Work out the finished part from the listing and answer in its coordinate system (mm). A direction names the side the tool comes from. Round coordinates to 2 decimals unless told otherwise and drop trailing zeros. Loops run counter-clockwise (first coordinate to the right, second up) from the corner with the lowest first, then second, coordinate; pieces in that order, holes last.
```python
from build123d import *

# Parameters (mm, degrees)
F0_R      = 23.300807
F1_DEPTH  = 76.2
F3_R      = 50.8
F3_R_2    = 23.300807
F4_DEPTH  = 12.7
F6_R      = 50.8
F6_R_2    = 23.300807
F7_DEPTH  = 12.7
F8_R      = 23.300807
F8_R_2    = 19.05
F9_DEPTH  = 12.7
F10_R     = 23.300807
F10_R_2   = 19.05
F11_DEPTH = 12.7
F12_R     = 6.35
F13_DEPTH = 2540


with BuildPart() as f1:
    # F0 (on Right) → F1 (new body)
    with BuildSketch(Plane.YZ):
        Circle(F0_R)
    extrude(amount=F1_DEPTH)



with BuildPart() as f4:
    # F3 (on face) → F4 (new body)
    with BuildSketch(Plane(origin=(0, 0, 0), x_dir=(0, -1, 0), z_dir=(-1, 0, 0))):
        Circle(F3_R)
        Circle(F3_R_2, mode=Mode.SUBTRACT)
    extrude(amount=F4_DEPTH)


with BuildPart() as f7:
    # F6 (on face) → F7 (new body)
    with BuildSketch(Plane.YZ.offset(76.2)):
        Circle(F6_R)
        Circle(F6_R_2, mode=Mode.SUBTRACT)
    extrude(amount=F7_DEPTH)


with BuildPart() as f1_1:
    add(f1.part)

    add(f7.part)  # F9 merges F7
    # F8 (on face) → F9 (join)
    with BuildSketch(Plane.YZ.offset(76.2)):
        Circle(F8_R)
        Circle(F8_R_2, mode=Mode.SUBTRACT)
    extrude(amount=F9_DEPTH)


    add(f4.part)  # F11 merges F4
    # F10 (on face) → F11 (join)
    with BuildSketch(Plane(origin=(0, 0, 0), x_dir=(0, -1, 0), z_dir=(-1, 0, 0))):
        Circle(F10_R)
        Circle(F10_R_2, mode=Mode.SUBTRACT)
    extrude(amount=F11_DEPTH)

    # F12 (on face) → F13 (cut)
    with BuildSketch(Plane(origin=(-12.7, 0, 0), x_dir=(0, -1, 0), z_dir=(-1, 0, 0))):
        with Locations((-38.1, 12.7)):
            Circle(F12_R)
        with Locations((-38.1, -12.7)):
            Circle(F12_R)
        with Locations((38.1, -12.7)):
            Circle(F12_R)
        with Locations((38.1, 12.7)):
            Circle(F12_R)
    extrude(amount=-F13_DEPTH, mode=Mode.SUBTRACT)


solid = f1_1.part
```
1. Find section B-B (z = 0). Write down the section's boundary in (x, y), then the cut area to 3 significant figures.
Answer key:
outline: (-12.7, -50.8) - (0, -50.8) - (0, -23.3) - (76.2, -23.3) - (76.2, -50.8) - (88.9, -50.8) - (88.9, -19.05) - (76.2, -19.05) - (76.2, 19.05) - (88.9, 19.05) - (88.9, 50.8) - (76.2, 50.8) - (76.2, 23.3) - (0, 23.3) - (0, 50.8) - (-12.7, 50.8) - (-12.7, 19.05) - (0, 19.05) - (0, -19.05) - (-12.7, -19.05) - close
area: 5,160 mm2
2. Given pin 1 (10 mm diameter, centred on y = 38.1, z = 12.7, fed in from -X); pin 2 (11.5 mm diameter, centred on y = 7, z = 7.5, fed in from +X); pin 3 (1.5 mm diameter, centred on x = 76, z = -14.5, fed in from +Y); pin 4 (19 mm diameter, centred on y = -0.5, z = 8.5, fed in from -X), each flat-ended and moving along its own axis, determine where each tip first touches the part or whether it passes through.
Answer key:
pin 1: passes through
pin 2: stops at x = 76.2
pin 3: stops at y = 48.9
pin 4: stops at x = 0
3. Find section C-C (y = 37). Write down the section's boundary in (x, z).
Answer key:
outline: (-12.7, -34.81) - (0, -34.81) - (0, -18.95) - (-12.7, -18.95) - close; (-12.7, -6.45) - (0, -6.45) - (0, 6.45) - (-12.7, 6.45) - close; (-12.7, 18.95) - (0, 18.95) - (0, 34.81) - (-12.7, 34.81) - close; (76.2, -34.81) - (88.9, -34.81) - (88.9, -18.95) - (76.2, -18.95) - close; (76.2, -6.45) - (88.9, -6.45) - (88.9, 6.45) - (76.2, 6.45) - close; (76.2, 18.95) - (88.9, 18.95) - (88.9, 34.81) - (76.2, 34.81) - close
4. Consider probe 1 along X at (y, z) = (-35.5, 34); probe 2 along Z at (x, y) = (-7.75, -38.1); probe 3 along Y at (x, z) = (86, 12). Determine where each line is inside the solid, lowest interval first.
Answer key:
probe 1: x = -12.7 to 0, 76.2 to 88.9
probe 2: z = -33.6 to -19.05, -6.35 to 6.35, 19.05 to 33.6
probe 3: y = -49.36 to -44.41, -31.79 to -14.8, 14.8 to 31.79, 44.41 to 49.36
5. Determine the mould class of faces 1 (the face through (-6.261, 11.012, -49.592)), 2 (the face through (82.461, 32.234, -15.132)), 3 (the face through (76.2, 11, -22)) for opening direction Y: +Y half, -Y half, draft (parallel to the pull), parting line (faces both ways), or undercut.
Answer key:
face 1: parting line
face 2: undercut
face 3: draft
6. Find section A-A (y = -30). Write down the section's boundary in (x, z), then the cut area to 3 significant figures.
Answer key:
outline: (-12.7, -41) - (0, -41) - (0, 41) - (-12.7, 41) - close; (76.2, -41) - (88.9, -41) - (88.9, 41) - (76.2, 41) - close
area: 2,080 mm2
7. Which of the six approach directions +Z, -Z, +X, -X, +Y, -Y give full straight-line access (tool end or side, diameter ignored) to faces 4 (the face through (-6.439, -31.756, 12.979)), 5 (the face through (37.57, -18.49, -14.18)), 6 (the face through (-6.26, 15.12, -11.59)), 7 (the face through (76.2, 0, 0))?
Answer key:
face 4: +X, -X
face 5: none
face 6: -X
face 7: +X
8. Find section D-D (z = -40). Write down the section's boundary in (x, y), then the cut area to 3 significant figures.
Answer key:
outline: (-12.7, -31.32) - (0, -31.32) - (0, 31.32) - (-12.7, 31.32) - close; (76.2, -31.32) - (88.9, -31.32) - (88.9, 31.32) - (76.2, 31.32) - close
area: 1,590 mm2
